```python
from build123d import *

# Parameters (mm, degrees)
EXTRUDE_1_DEPTH  = 115
FILLET_5_R       = 2.5
FILLET_6_R       = 2.5
FILLET_8_R       = 2.5
FILLET_10_R      = 2.5
FILLET_11_R      = 2.5
EXTRUDE_2_DEPTH  = 5
EXTRUDE_3_DEPTH  = 5
FILLET_12_R      = 10
CHAMFER_2_SIZE   = 5.361267301
CHAMFER_2_SIZE_2 = 2.5
EXTRUDE_5_DEPTH  = 5
FILLET_13_R      = 15


# Some blends are built 0.0001 mm under size
with BuildPart() as part:
    # ｽｹｯﾁ1 → ﾎﾞｽ - 押し出し1 (new body)
    with BuildSketch(Plane(origin=(0, 0, 0), x_dir=(1, 0, 0), z_dir=(0, 1, 0))):
        Polygon((47.807009209, -4.786582838), (36.65910681, -31.7), (5, -31.7), (5, 36.7), (-26, 36.7), (-26, 16.7), (-21, 16.7), (-21, 31.7), (0, 31.7), (0, -36.7), (40, -36.7), (52.426406871, -6.7), align=None)
    extrude(amount=EXTRUDE_1_DEPTH)

    # ﾌｨﾚｯﾄ5
    fillet_5_edges = [part.edges().sort_by_distance(p)[0] for p in [
        (-26, 57.5, -36.7),
    ]]
    fillet(fillet_5_edges, radius=FILLET_5_R)

    # ﾌｨﾚｯﾄ6
    fillet_6_edges = [part.edges().sort_by_distance(p)[0] for p in [
        (5, 57.5, -36.7),
    ]]
    fillet(fillet_6_edges, radius=FILLET_6_R)

    # ﾌｨﾚｯﾄ8
    fillet_8_edges = [part.edges().sort_by_distance(p)[0] for p in [
        (52.426406871, 57.5, 6.7),
        (47.807009209, 57.5, 4.786582838),
    ]]
    fillet(fillet_8_edges, radius=FILLET_8_R - 0.0001)  # a hair under: the kernel refuses the full size

    # ﾌｨﾚｯﾄ10
    fillet_10_edges = [part.edges().sort_by_distance(p)[0] for p in [
        (0, 57.5, 36.7),
    ]]
    fillet(fillet_10_edges, radius=FILLET_10_R)

    # ﾌｨﾚｯﾄ11
    fillet_11_edges = [part.edges().sort_by_distance(p)[0] for p in [
        (5, 57.5, 31.7),
    ]]
    fillet(fillet_11_edges, radius=FILLET_11_R)

    # ｽｹｯﾁ2 → ﾎﾞｽ - 押し出し2 (add)
    with BuildSketch(Plane(origin=(0, 115, 0), x_dir=(1, 0, 0), z_dir=(0, 1, 0))):
        with BuildLine():
            Line((49.159999459, -5.55299025), (40, -5.55299025))
            Line((40, -5.55299025), (5, -5.55299025))
            Line((5, -5.55299025), (5, -36.7))
            Line((5, -36.7), (40, -36.7))
            Line((40, -36.7), (51.46969829, -9.009698831))
            ThreePointArc((51.46969829, -9.009698831), (51.23867349, -6.664064668), (49.159999459, -5.55299025))
        make_face()
    extrude(amount=-EXTRUDE_2_DEPTH)

    # ｽｹｯﾁ3 → ﾎﾞｽ - 押し出し3 (add)
    with BuildSketch(Plane(origin=(0, 0, -36.7), x_dir=(-1, 0, 0), z_dir=(0, 0, -1))):
        with BuildLine():
            Line((6.851817904, 90), (-51.659999459, 90))
            Line((-51.659999459, 90), (-61.659999459, 90))
            Line((-61.659999459, 90), (-61.659999459, 85))
            ThreePointArc((-61.659999459, 85), (-51.659999459, 75), (-61.659999459, 65))
            Line((-61.659999459, 65), (-61.659999459, 60))
            Line((-61.659999459, 60), (-51.659999459, 60))
            Line((-51.659999459, 60), (6.851817904, 60))
            Line((6.851817904, 60), (6.851817904, 90))
        make_face()
    extrude(amount=-EXTRUDE_3_DEPTH)

    # ﾌｨﾚｯﾄ12
    fillet_12_edges = [part.edges().sort_by_distance(p)[0] for p in [
        (5, 75, -31.7),
    ]]
    fillet(fillet_12_edges, radius=FILLET_12_R)

    # 面取り2
    # the kernel refuses this chamfer: 5.361267301, 2.5 mm, written as the material it takes off along each edge
    with BuildSketch(Plane(origin=(61.659999459, 75, -36.7), x_dir=(0.9839382263976153, 0.1785092900482071, 0), z_dir=(0.1785092900482071, -0.9839382263976153, 0))) as chamfer_2_piece_1:
        Polygon((10, CHAMFER_2_SIZE), (10 + CHAMFER_2_SIZE_2, 0), (10, 0), align=None)
    revolve(axis=Axis((61.659999459, 75, -36.7), (0, 0, 1)), revolution_arc=339.434115604, mode=Mode.SUBTRACT)

    # ｽｹｯﾁ4 → ﾎﾞｽ - 押し出し5 (add)
    with BuildSketch(Plane(origin=(0, 0, 5.55299025), x_dir=(-1, 0, 0), z_dir=(0, 0, -1))):
        with BuildLine():
            Line((-46.850300628, 90), (-51.659999459, 90))
            Line((-51.659999459, 90), (-61.659999459, 90))
            Line((-61.659999459, 90), (-61.659999459, 85))
            ThreePointArc((-61.659999459, 85), (-51.659999459, 75), (-61.659999459, 65))
            Line((-61.659999459, 65), (-61.659999459, 60))
            Line((-61.659999459, 60), (-51.659999459, 60))
            Line((-51.659999459, 60), (-46.850300628, 60))
            Line((-46.850300628, 60), (-46.850300628, 90))
        make_face()
    extrude(amount=-EXTRUDE_5_DEPTH)

    # ﾌｨﾚｯﾄ13
    # the kernel refuses this fillet: 15 mm, written as the material it adds along each edge
    with BuildSketch(Plane(origin=(50.830446054, 90, 10.55299025), x_dir=(-0.3826834323650874, 0, 0.9238795325112876), z_dir=(0, -1, 0))) as fillet_13_piece_1_section:
        with BuildLine():
            CenterArc((FILLET_13_R * 0.668178637919, -FILLET_13_R), FILLET_13_R, 90, 67.5)
            Line((-FILLET_13_R * 0.255700894592, -FILLET_13_R * 0.617316567635), (0, 0))
            Line((0, 0), (FILLET_13_R * 0.668178637919, 0))
        make_face()
    fillet_13_piece_1 = extrude(amount=30, mode=Mode.PRIVATE)
    fillet_13_piece_1 = fillet_13_piece_1 - Plane(origin=(61.659999459, 75, 12.967680369), x_dir=(0, 1, 0), z_dir=(0, 0, -1)) * Cylinder(10, 101, mode=Mode.PRIVATE)
    add(fillet_13_piece_1)


solid = part.part
```
Model file for the job. Use its own axes, mm. A direction names the side the tool comes from. Coordinates: 2 decimals unless noted, no trailing zeros. Loops run counter-clockwise (first coordinate to the right, second up) from the corner with the lowest first, then second, coordinate; pieces in that order, holes last. Notation, with made-up numbers: (-3.75, -39) -> (45.25, -39) arc R20 ccw to (45.25, -27) -> close; hole circle Ø6 at (73.25, 46). An arc over 180 degrees is marked (long way). Answer as a JSON object with one key per item and string values.
Q1. Flat gauge pins, fed straight in: P1, Ø12, axis at y = 100, z = -1.5, coming from the +X side; P2, Ø6.5, axis at x = -10, y = 63.5, coming from the +Z side; P3, Ø1.5, axis at x = 16, y = 112, coming from the -Z side; P4, Ø12, axis at x = 50.5, z = -2.5, coming from the -Y side. Where does each tip first touch, or does it go through?
Report:
{"P1": "stops at x = 5", "P2": "stops at z = -31.7", "P3": "stops at z = 5.55", "P4": "passes through"}
Q2. Probe probe 1 along Z at (x, y) = (15, 83); probe 2 along X at (y, z) = (68, -22); probe 3 along Z at (x, y) = (18, 38). List the from-to ranges inside material, lowest first.
Report:
{"probe 1": "z = -36.7 to -31.7, 31.7 to 36.7", "probe 2": "x = -26 to -21, 0 to 5", "probe 3": "z = 31.7 to 36.7"}
Q3. 3-axis set-ups, long thin cutter, end or side, ignore diameter. For faces 1 (the flat face through (25, 90, -34)), 2 (the cylindrical face through (4.248, 30.42, -35.987)), 3 (the cylindrical face through (7.85, 74.79, -28.69)), 4 (the flat face through (-24, 57, -16.7)), 5 (the flat face through (22, 54, 31.7)): which of +Z, -Z, +X, -X, +Y, -Y reach the whole face in a straight line?
Report:
{"face 1": "-Z, +X, +Y", "face 2": "-Z, +X, -Y", "face 3": "+X, +Y, -Y", "face 4": "+Z, -X, +Y, -Y", "face 5": "-Y"}
Q4. Cut at A-A (x = 29). List the corners of the cut face in (y, z), and give its area (3 significant figures).
Report:
{"outline": "(0, 31.7) -> (110, 31.7) -> (110, 5.55) -> (115, 5.55) -> (115, 36.7) -> (0, 36.7) -> close; (60, -36.7) -> (90, -36.7) -> (90, -31.7) -> (60, -31.7) -> close", "area": "856 mm2"}
Q5. Cut at C-C (x = -18). List the corners of the cut face in (y, z).
Report:
{"outline": "(0, -36.7) -> (115, -36.7) -> (115, -31.7) -> (0, -31.7) -> close"}
Q6. Pull direction X, two halves, no side cores. Call faces 6 (the flat face through (51, 75, 5.553)), 7 (the cylindrical face through (0.752, 58.305, 35.987)), 8 (the cylindrical face through (48.178, 58.305, 5.754)): released by +X, released by -X, zero draft, split by the parting line, or undercut.
Report:
{"face 6": "zero draft", "face 7": "released by -X", "face 8": "undercut"}
Q7. Cut at D-D (z = 0.5). List the corners of the cut face in (x, y), and give its area (3 significant figures).
Report:
{"outline": "(0, 0) -> (5, 0) -> (5, 115) -> (0, 115) -> close", "area": "575 mm2"}
